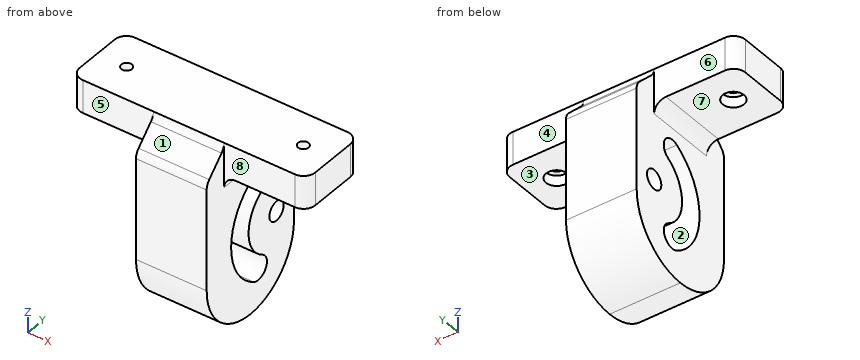
from build123d import *

# Parameters (mm, degrees)
SKETCH1_W               = 100
SKETCH1_H               = 30
BOSS_EXTRUDE1_DEPTH     = 14
SKETCH2_R               = 2.25
CUT_EXTRUDE1_DEPTH      = 14
SKETCH3_R               = 4.5
CUT_EXTRUDE2_DEPTH      = 4.4
BOSS_EXTRUDE2_DEPTH     = 15
CUT_EXTRUDE3_DEPTH      = 116.485929879
CUT_EXTRUDE3_DEPTH_BACK = 116.485929879
SKETCH6_R               = 4.1
FILLET1_R               = 25
CUT_EXTRUDE5_DEPTH      = 116.485929879
CUT_EXTRUDE5_DEPTH_BACK = 116.485929879
FILLET2_R               = 5


# Some blends are built 0.0001 mm under size
with BuildPart() as part:
    # Sketch1 → Boss-Extrude1 (new body)
    with BuildSketch(Plane(origin=(0, 0, -7), x_dir=(-1, 0, 0), z_dir=(0, 0, -1))):
        with Locations((0, -29)):
            Rectangle(SKETCH1_W, SKETCH1_H)
    extrude(amount=BOSS_EXTRUDE1_DEPTH)

    # Sketch2 → Cut-Extrude1 (cut)
    with BuildSketch(Plane(origin=(0, 0, -21), x_dir=(-1, 0, 0), z_dir=(0, 0, -1))):
        with Locations((-37.5, -29)):
            Circle(SKETCH2_R)
        with Locations((37.5, -29)):
            Circle(SKETCH2_R)
    extrude(amount=-CUT_EXTRUDE1_DEPTH, mode=Mode.SUBTRACT)

    # Sketch3 → Cut-Extrude2 (cut)
    with BuildSketch(Plane(origin=(0, 0, -21), x_dir=(-1, 0, 0), z_dir=(0, 0, -1))):
        with Locations((-37.5, -29)):
            Circle(SKETCH3_R)
        with Locations((37.5, -29)):
            Circle(SKETCH3_R)
    extrude(amount=-CUT_EXTRUDE2_DEPTH, mode=Mode.SUBTRACT)

    # Sketch5 → Boss-Extrude2 (add, symmetric)
    with BuildSketch(Plane(origin=(0, 0, 0), x_dir=(0, 0, -1), z_dir=(1, 0, 0))):
        Polygon((9, -14), (19, -4), (89, -4), (89, -54), (19, -54), (9, -44), align=None)
    extrude(amount=BOSS_EXTRUDE2_DEPTH, both=True)

    # Sketch6 → Cut-Extrude3 (cut, two sides: drawn at the far end of the back side and taken through both)
    with BuildSketch(Plane(origin=(0, 0, 0), x_dir=(0, 0, -1), z_dir=(1, 0, 0)).offset(-CUT_EXTRUDE3_DEPTH_BACK)):
        with Locations((54, -14)):
            Circle(SKETCH6_R)
    extrude(amount=CUT_EXTRUDE3_DEPTH + CUT_EXTRUDE3_DEPTH_BACK, mode=Mode.SUBTRACT)

    # Fillet1
    fillet1_edges = [part.edges().sort_by_distance(p)[0] for p in [
        (0, -4, -89),
        (0, -54, -89),
    ]]
    fillet(fillet1_edges, radius=FILLET1_R - 0.0001)  # a hair under: the kernel refuses the full size

    # Sketch7 → Cut-Extrude5 (cut, two sides: drawn at the far end of the back side and taken through both)
    with BuildSketch(Plane(origin=(0, 0, 0), x_dir=(0, 0, -1), z_dir=(1, 0, 0)).offset(-CUT_EXTRUDE5_DEPTH_BACK)):
        with BuildLine():
            ThreePointArc((31.483339502, -27), (54, -40), (76.516660498, -27))
            ThreePointArc((76.516660498, -27), (74.686533479, -20.169872981), (67.856406461, -22))
            ThreePointArc((67.856406461, -22), (54, -30), (40.143593539, -22))
            ThreePointArc((40.143593539, -22), (33.313466521, -20.169872981), (31.483339502, -27))
        make_face()
    extrude(amount=CUT_EXTRUDE5_DEPTH + CUT_EXTRUDE5_DEPTH_BACK, mode=Mode.SUBTRACT)

    # Fillet2
    # the kernel refuses this fillet: 5 mm, written as the material it adds along each edge
    with BuildSketch(Plane(origin=(-15, -14, -21), x_dir=(0, 0, -1), z_dir=(0, -1, 0))) as fillet2_piece_1:
        with BuildLine():
            CenterArc((FILLET2_R, -FILLET2_R), FILLET2_R, 90, 90)
            Line((0, -FILLET2_R), (0, 0))
            Line((0, 0), (FILLET2_R, 0))
        make_face()
    extrude(amount=30)
    with BuildSketch(Plane(origin=(15, -14, -21), x_dir=(0, 0, -1), z_dir=(0, -1, 0))) as fillet2_piece_2:
        with BuildLine():
            CenterArc((FILLET2_R, FILLET2_R), FILLET2_R, 180, 90)
            Line((0, FILLET2_R), (0, 0))
            Line((0, 0), (FILLET2_R, 0))
        make_face()
    extrude(amount=30)
    with BuildSketch(Plane(origin=(-15, -14, -9), x_dir=(0, 0.707106781186544, -0.7071067811865509), z_dir=(1, 0, 0))) as fillet2_piece_3_section:
        with BuildLine():
            CenterArc((FILLET2_R * 0.414213562373, FILLET2_R), FILLET2_R, 225, 45)
            Line((-FILLET2_R * 0.292893218813, FILLET2_R * 0.292893218813), (0, 0))
            Line((0, 0), (FILLET2_R * 0.414213562373, 0))
        make_face()
    fillet2_piece_3 = extrude(amount=30, mode=Mode.PRIVATE)
    fillet2_piece_3 = split(fillet2_piece_3, bisect_by=Plane(origin=(0, -13.688256851, -7), z_dir=(0, 0, -1)), keep=Keep.TOP, mode=Mode.PRIVATE)
    add(fillet2_piece_3)
    with BuildSketch(Plane(origin=(-15, -44, -9), x_dir=(0, -0.707106781186544, -0.7071067811865509), z_dir=(1, 0, 0))) as fillet2_piece_4_section:
        with BuildLine():
            CenterArc((FILLET2_R * 0.414213562373, -FILLET2_R), FILLET2_R, 90, 45)
            Line((-FILLET2_R * 0.292893218813, -FILLET2_R * 0.292893218813), (0, 0))
            Line((0, 0), (FILLET2_R * 0.414213562373, 0))
        make_face()
    fillet2_piece_4 = extrude(amount=30, mode=Mode.PRIVATE)
    fillet2_piece_4 = split(fillet2_piece_4, bisect_by=Plane(origin=(0, -44.311743149, -7), z_dir=(0, 0, -1)), keep=Keep.TOP, mode=Mode.PRIVATE)
    add(fillet2_piece_4)
    # the kernel refuses this fillet: 5 mm, written as the material it takes off along each edge
    with BuildSketch(Plane(origin=(-20.17766953, -54, -19), x_dir=(0, 0, -1), z_dir=(1, 0, 0))) as fillet2_2_piece_1:
        with BuildLine():
            CenterArc((FILLET2_R * 0.414213562373, FILLET2_R), FILLET2_R, 225, 45)
            Line((-FILLET2_R * 0.292893218813, FILLET2_R * 0.292893218813), (0, 0))
            Line((0, 0), (FILLET2_R * 0.414213562373, 0))
        make_face()
    extrude(amount=40.355339059, mode=Mode.SUBTRACT)
    with BuildSketch(Plane(origin=(20.17766953, -4, -19), x_dir=(0, -0.7071067811865441, 0.707106781186551), z_dir=(-1, 0, 0))) as fillet2_2_piece_2:
        with BuildLine():
            CenterArc((FILLET2_R * 0.414213562373, -FILLET2_R), FILLET2_R, 90, 45)
            Line((-FILLET2_R * 0.292893218813, -FILLET2_R * 0.292893218813), (0, 0))
            Line((0, 0), (FILLET2_R * 0.414213562373, 0))
        make_face()
    extrude(amount=40.355339059, mode=Mode.SUBTRACT)
    with BuildSketch(Plane(origin=(50, -14, 5.5), x_dir=(-1, 0, 0), z_dir=(0, 0, -1)), Plane(origin=(50, -44, 5.5), x_dir=(0, 1, 0), z_dir=(0, 0, -1))) as fillet2_2_piece_3:
        with BuildLine():
            CenterArc((FILLET2_R, -FILLET2_R), FILLET2_R, 90, 90)
            Line((0, -FILLET2_R), (0, 0))
            Line((0, 0), (FILLET2_R, 0))
        make_face()
    extrude(amount=39, mode=Mode.SUBTRACT)
    with BuildSketch(Plane(origin=(-50, -14, 5.5), x_dir=(1, 0, 0), z_dir=(0, 0, -1)), Plane(origin=(-50, -44, 5.5), x_dir=(0, 1, 0), z_dir=(0, 0, -1))) as fillet2_2_piece_4:
        with BuildLine():
            CenterArc((FILLET2_R, FILLET2_R), FILLET2_R, 180, 90)
            Line((0, FILLET2_R), (0, 0))
            Line((0, 0), (FILLET2_R, 0))
        make_face()
    extrude(amount=39, mode=Mode.SUBTRACT)


solid = part.part
Verification items for the finished model (mm, model axes). Face numbers are marked on the shaded views. A direction names the side the tool comes from. Round coordinates to 2 decimals unless told otherwise and drop trailing zeros. Loops run counter-clockwise (first coordinate to the right, second up) from the corner with the lowest first, then second, coordinate; pieces in that order, holes last. Notation, with made-up numbers: (-33, 3) - (26, 3) arc R22 cw to (26, 32) - close; hole circle Ø11 at (-26.5, 20). An arc over 180 degrees is marked (long way). Answer in a Markdown table with one row per item. Add a question column.
Q1. Gauge pin test, flat ends, axial feed: pin 1 (4 mm diameter, centred on x = -37.5, y = -29, fed in from -Z); pin 2 (9 mm diameter, centred on x = -31, y = -26, fed in from -Z); pin 3 (21 mm diameter, centred on x = -27.5, z = -20.5, fed in from -Y); pin 4 (8 mm diameter, centred on x = 37.5, y = -29, fed in from -Z). Record the tip position at first contact, or that the pin passes through.
Q2. Section check A-A on x = 10. State how many separate pieces and enclosed holes the cut face has, plus the area to 3 significant figures.
Q3. Section check B-B on z = -43. Enter the section's corners in (x, y), plus the area to 3 significant figures.
Q4. Tool access check on the marked faces 4, 5, 6, 7 and 8. Record the directions out of +Z, -Z, +X, -X, +Y, -Y that give a thin tool (end or side, any length) a straight path to the whole face; none if there is none.
Q5. Release check for a two-part mould opening along Y. For the marked faces 1, 2 and 3 record: pulls with the +Y half, pulls with the -Y half, needs draft (parallel to the pull), parting line crosses it, or undercut.
Q6. Material ranges on line 1 (Z direction, x = 25, y = -29); line 2 (X direction, y = -41, z = -64.5); line 3 (Z direction, x = 4, y = -36), recorded low to high.
Q7. Section check D-D on z = -54. Enter the section's corners in (x, y), plus the area to 3 significant figures.
Q8. Section check C-C on x = -37.5. Enter the section's corners in (y, z).
Found:
| question | item | result |
|---|---|---|
| 1 | pin 1 | passes through |
| 1 | pin 2 | stops at z = -21 |
| 1 | pin 3 | stops at y = -44 |
| 1 | pin 4 | stops at z = -16.6 |
| 2 | separate pieces | 1 |
| 2 | enclosed holes | 2 |
| 2 | area | 3,120 mm² |
| 3 | outline | (-15, -54) - (15, -54) - (15, -37.56) - (-15, -37.56) - close; (-15, -25.62) - (15, -25.62) - (15, -4) - (-15, -4) - close |
| 3 | area | 1,140 mm² |
| 4 | face 4 | +Z, -Z, +X, +Y |
| 4 | face 5 | +Z, -Z, -X, -Y |
| 4 | face 6 | +Z, -Z, -X, +Y |
| 4 | face 7 | -Z, -X, +Y, -Y |
| 4 | face 8 | +Z, -Z, +X, -Y |
| 5 | face 1 | pulls with the -Y half |
| 5 | face 2 | undercut |
| 5 | face 3 | needs draft |
| 6 | line 1 | z = -21 to -7 |
| 6 | line 2 | x = -15 to 15 |
| 6 | line 3 | z = -88 to -67.86, -40.14 to -7 |
| 7 | outline | (-15, -54) - (15, -54) - (15, -40) - (-15, -40) - close; (-15, -30) - (15, -30) - (15, -18.1) - (-15, -18.1) - close; (-15, -9.9) - (15, -9.9) - (15, -4) - (-15, -4) - close |
| 7 | area | 954 mm² |
| 8 | outline | (-44, -21) - (-33.5, -21) - (-33.5, -16.6) - (-31.25, -16.6) - (-31.25, -7) - (-44, -7) - close; (-26.75, -16.6) - (-24.5, -16.6) - (-24.5, -21) - (-14, -21) - (-14, -7) - (-26.75, -7) - close |
